The model under review builds one solid part; all positions refer to its coordinate system, in mm. Face numbers are marked on the shaded views. Round coordinates to 2 decimals unless told otherwise and drop trailing zeros. Order: outer loops, then holes, each group sorted by start corner. A loop starts at its lowest first (then second) coordinate and runs counter-clockwise, first axis right, second up. Notation, with made-up numbers: (2, -23) -> (27, -23) arc R16 ccw to (27, -2) -> close; hole circle Ø9 at (67.25, -0.75). An arc over 180 degrees is marked (long way). Use a Markdown table: item, result. Add a question column.
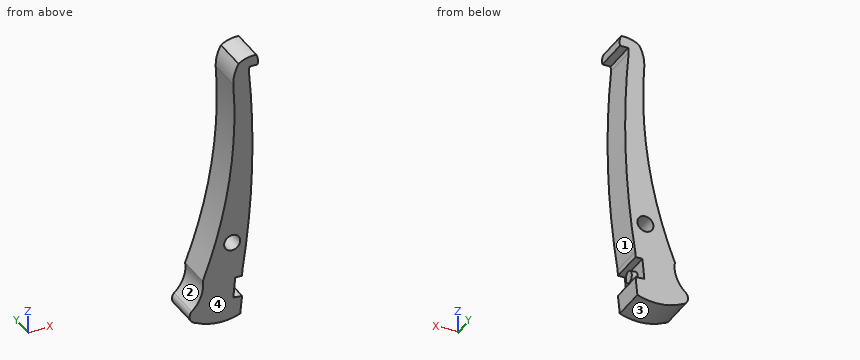
```python
from build123d import *

# Parameters (mm, degrees)
F1_DEPTH = 3.81
F4_D     = 1.778
F5_R     = 0.6352589674
F6_DEPTH = 0.635


# Not quite as in the source:
# - a feature of the source that left no trace in its solid (it failed there, or was rolled back) is left out
# - a feature names something its author has since deleted; it is built from what else it names


with BuildPart() as f1:
    # F0 (on Front) → F1 (new body)
    with BuildSketch(Plane.XZ):
        with BuildLine():
            ThreePointArc((-31.4986416626, 9.8449740097), (-31.6959768892, 8.9855931424), (-31.0501495083, 8.3852735102))
            ThreePointArc((-31.0501495083, 8.3852735102), (-28.6350189428, 7.6831870892), (-26.1434996057, 8.026861912))
            Line((-26.1434996057, 8.026861912), (-25.9436036256, 10.0525402048))
            Line((-25.9436036256, 10.0525402048), (-26.9064083695, 10.1394830272))
            Line((-26.9064083695, 10.1394830272), (-26.7011658463, 12.4123385609))
            Line((-26.7011658463, 12.4123385609), (-25.9436036256, 12.4123385609))
            Line((-25.9436036256, 12.4123385609), (-25.9087286158, 13.0410402551))
            ThreePointArc((-25.9087286158, 13.0410402551), (-24.8435996749, 24.5554030542), (-25.1834829825, 36.1139293298))
            Line((-25.1834829825, 36.1139293298), (-25.1380671304, 36.6562315202))
            Line((-25.1380671304, 36.6562315202), (-24.2339836005, 36.6562315202))
            ThreePointArc((-24.2339836005, 36.6562315202), (-24.1923341682, 37.2519069884), (-24.3619682602, 37.8244349033))
            ThreePointArc((-24.3619682602, 37.8244349033), (-25.3896581056, 37.7581269753), (-26.3316547054, 37.3419712767))
            ThreePointArc((-26.3316547054, 37.3419712767), (-26.7797456815, 36.2582545781), (-26.9143641051, 35.0933059588))
            ThreePointArc((-26.9143641051, 35.0933059588), (-27.3654380994, 23.8788044049), (-30.282865234, 13.0410402552))
            ThreePointArc((-30.282865234, 13.0410402552), (-30.4786310467, 11.2862366956), (-31.4986416626, 9.8449740097))
        make_face()
    extrude(amount=F1_DEPTH)

    # F4 (through all)
    with Locations(Plane(origin=(0, 0, 0), x_dir=(1, 0, 0), z_dir=(0, 1, 0))):
        with Locations((-27.0313583314, -16.6009981185)):
            Hole(F4_D / 2)

    # F5 (on face) → F6 (join)
    with BuildSketch(Plane(origin=(-27.5969837191, 0, 2.4920521733), x_dir=(0, 1, 0), z_dir=(0.9959475762, 0, -0.0899356737))):
        with Locations((-1.905, 8.8195993749)):
            Circle(F5_R)
    extrude(amount=F6_DEPTH)


solid = f1.part
```
Q1. Add section D-D, the plane y = -1.95. Give the boundary of the cut face in (x, z), then the cut area to 3 significant figures.
Q2. Add section A-A, the plane z = 16. Give the boundary of the cut face in (x, y), then the cut area to 3 significant figures.
Q3. For pin 1 (1 mm diameter, centred on y = -2, z = 34.5, fed in from +X); pin 2 (2 mm diameter, centred on x = -27.03, z = 16.6, fed in from +Y); pin 3 (0.6 mm diameter, centred on x = -26.5, y = -1, fed in from -Z); pin 4 (0.5 mm diameter, centred on x = -24.5, y = -3, fed in from -Z), all flat-tipped, find the tip position at first contact; note any pin that passes through.
Q4. Add section C-C, the plane y = -3.3. Give the boundary of the cut face in (x, z).
Q5. Add section B-B, the plane x = -27.25. Give the boundary of the cut face in (y, z), then the cut area to 3 significant figures.
Q6. To check wall thickness, follow line 1 along Z through (x, y) = (-26.5, -0.3); line 2 along Z through (x, y) = (-26.25, -3.45); line 3 along X through (y, z) = (-3.2, 35.5). State the ranges of each line that lie inside material, in increasing order.
Q7. Draft analysis for pull direction Z (two halves, no side actions). For the marked faces 1, 2, 3 and 4, state which applies: released by +Z, released by -Z, zero draft, split by the parting line, or undercut.
Return value:
| question | item | result |
|---|---|---|
| 1 | outline | (-31.5, 9.84) arc R0.88 ccw to (-31.05, 8.39) arc R6.03 ccw to (-26.14, 8.03) -> (-25.94, 10.05) -> (-26.91, 10.14) -> (-26.86, 10.64) -> (-26.23, 10.59) -> (-26.11, 11.85) -> (-26.75, 11.91) -> (-26.7, 12.41) -> (-25.94, 12.41) -> (-25.91, 13.04) arc R95.12 ccw to (-25.18, 36.11) -> (-25.14, 36.66) -> (-24.23, 36.66) arc R1.68 ccw to (-24.36, 37.82) arc R2.94 ccw to (-26.33, 37.34) arc R4.25 ccw to (-26.91, 35.09) arc R50.49 cw to (-30.28, 13.04) arc R3.54 cw to start; hole circle Ø1.78 at (-27.03, 16.6) |
| 1 | area | 86.0 mm² |
| 2 | outline | (-29.23, -3.81) -> (-27.69, -3.81) -> (-27.69, 0) -> (-29.23, 0) -> close; (-26.38, -3.81) -> (-25.5, -3.81) -> (-25.5, 0) -> (-26.38, 0) -> close |
| 2 | area | 9.20 mm² |
| 3 | pin 1 | x = -25.02 |
| 3 | pin 2 | y = 0 |
| 3 | pin 3 | z = 7.83 |
| 3 | pin 4 | z = 36.66 |
| 4 | outline | (-31.5, 9.84) arc R0.88 ccw to (-31.05, 8.39) arc R6.03 ccw to (-26.14, 8.03) -> (-25.94, 10.05) -> (-26.91, 10.14) -> (-26.7, 12.41) -> (-25.94, 12.41) -> (-25.91, 13.04) arc R95.12 ccw to (-25.18, 36.11) -> (-25.14, 36.66) -> (-24.23, 36.66) arc R1.68 ccw to (-24.36, 37.82) arc R2.94 ccw to (-26.33, 37.34) arc R4.25 ccw to (-26.91, 35.09) arc R50.49 cw to (-30.28, 13.04) arc R3.54 cw to start; hole circle Ø1.78 at (-27.03, 16.6) |
| 5 | outline | (-3.81, 7.74) -> (0, 7.74) -> (0, 15.74) -> (-3.81, 15.74) -> close; (-3.81, 17.46) -> (0, 17.46) -> (0, 24.68) -> (-3.81, 24.68) -> close |
| 5 | area | 58.0 mm² |
| 6 | line 1 | 7.91 to 10.1, 12.41 to 15.89, 17.31 to 37.03 |
| 6 | line 2 | 7.99 to 10.08, 12.41 to 16.18, 17.03 to 37.39 |
| 6 | line 3 | -26.9 to -25.13 |
| 7 | face 1 | undercut |
| 7 | face 2 | undercut |
| 7 | face 3 | released by -Z |
| 7 | face 4 | zero draft |
